For this review, take the finished solid that the model builds, in its own axes (mm). A direction names the side the tool comes from. Round coordinates to 2 decimals unless told otherwise and drop trailing zeros. Write each loop counter-clockwise with the first axis right and the second up, starting at its lowest first coordinate (ties: lowest second). Pieces come first, ordered by that corner, then holes.
Autodesk Inventor part; units mm, degrees
ref_plane "YZ Plane" through (0, 0, 0) normal (1, 0, 0) x (0, 1, 0)
ref_plane "XZ Plane" through (0, 0, 0) normal (0, 1, 0) x (-1, 0, 0)
ref_plane "XY Plane" through (0, 0, 0) normal (0, 0, 1) x (1, 0, 0)
sketch "Sketch1" plane through (0, 0, 0) normal (0, 1, 0) x (-1, 0, 0)
  line L0 (-71.934, -191.4381) -> (-71.9231, -191.4456)
  line L1 (19.6087, -153.4475) -> (19.6065, -153.4456)
  line L2 (-67.3897, -0.1562) -> (-37.3897, -0.1562)
  line L3 (-37.3897, 1.8438) -> (-67.3897, 1.8438)
  line L4 (-62.3897, -3.1562) -> (-42.3897, -3.1562)
  line L5 (-42.3897, -5.1562) -> (-62.3897, -5.1562)
  line L6 (-113.9275, -186.1817) -> (-113.9275, -186.2664)
  line L7 (-115.4443, -311.1974) -> (-115.4443, -311.1982)
  line L8 (-113.9275, -180.4456) -> (-113.9275, -180.5089)
  circle A0 centre (-110.3897, -10.1562) radius 3
  arc A1 (10.8743, -2.1562) -> (10.8743, -18.1562) centre (10.8743, -10.1562) ccw
  arc A2 (-42.3897, -5.1562) -> (-42.3897, -3.1562) centre (-42.3897, -4.1562) ccw
  arc A3 (-62.3897, -3.1562) -> (-62.3897, -5.1562) centre (-62.3897, -4.1562) ccw
  arc A4 (-67.3897, 1.8438) -> (-67.3897, -0.1562) centre (-67.3897, 0.8438) ccw
  arc A5 (-37.3897, -0.1562) -> (-37.3897, 1.8438) centre (-37.3897, 0.8438) ccw
  arc A6 (-104.3897, 9.8438) -> (-104.3897, -30.1562) centre (-104.3897, -10.1562) ccw
  line L9 (5.6103, 9.8438) -> (11.6725, 6.3438)
  line L10 (11.6725, 6.3438) -> (15.6725, 6.3438)
  line L11 (15.6725, 6.3438) -> (15.6725, -0.2278)
  line L12 (15.6725, -0.2278) -> (13.3743, -2.1562)
  line L13 (13.3743, -2.1562) -> (10.8743, -2.1562)
  line L14 (5.6103, 9.8438) -> (-104.3897, 9.8438)
  line L15 (-89.3897, 0.552) -> (-101.3897, 0.552)
  line L16 (-101.3897, 0.552) -> (-95.3897, -6.1562)
  line L17 (-95.3897, -6.1562) -> (-89.3897, 0.552)
  line L18 (-85.3897, -4.1562) -> (-81.3897, -0.1562)
  line L19 (-75.3897, -0.1562) -> (-71.3897, -4.1562)
  line L20 (-71.3897, -4.1562) -> (-85.3897, -4.1562)
  line L21 (-81.3897, -0.1562) -> (-75.3897, -0.1562)
  line L22 (-68.2196, -182.5089) -> (-68.232, -182.5206)
  line L23 (-104.3897, 9.8438) -> (-104.3897, -30.1562)
  line L24 (-104.3897, -10.1562) -> (10.8743, -10.1562)
  line L25 (-110.3897, -10.1562) -> (-104.3897, -10.1562)
  line L26 (10.8743, -2.1562) -> (10.8743, -18.1562)
  line L27 (5.6103, -30.1562) -> (11.6725, -26.6562)
  line L28 (11.6725, -26.6562) -> (15.6725, -26.6562)
  line L29 (15.6725, -26.6562) -> (15.6725, -20.0845)
  line L30 (15.6725, -20.0845) -> (13.3743, -18.1562)
  line L31 (13.3743, -18.1562) -> (10.8743, -18.1562)
  line L32 (5.6103, -30.1562) -> (-104.3897, -30.1562)
  line L33 (-2.3577, 2.8438) -> (-7.5577, 2.8438)
  line L34 (-7.5577, 2.8438) -> (-7.5577, 4.8438)
  line L35 (-2.3577, 4.8438) -> (-7.5577, 4.8438)
  line L36 (-2.3577, 2.8438) -> (-2.3577, 4.8438)
  line L37 (-12.3577, 2.8438) -> (-17.5577, 2.8438)
  line L38 (-17.5577, 2.8438) -> (-17.5577, 4.8438)
  line L39 (-12.3577, 4.8438) -> (-17.5577, 4.8438)
  line L40 (-12.3577, 2.8438) -> (-12.3577, 4.8438)
  line L41 (-46.7577, -10.1562) -> (-46.7577, 9.8438)
  line L42 (-2.3577, -23.1562) -> (-7.5577, -23.1562)
  line L43 (-7.5577, -23.1562) -> (-7.5577, -25.1562)
  line L44 (-2.3577, -25.1562) -> (-7.5577, -25.1562)
  line L45 (-2.3577, -23.1562) -> (-2.3577, -25.1562)
  line L46 (-12.3577, -23.1562) -> (-17.5577, -23.1562)
  line L47 (-17.5577, -23.1562) -> (-17.5577, -25.1562)
  line L48 (-12.3577, -25.1562) -> (-17.5577, -25.1562)
  line L49 (-12.3577, -23.1562) -> (-12.3577, -25.1562)
  circle A7 centre (3.6423, -25.1562) radius 1.55
  circle A8 centre (3.5423, 4.8438) radius 1.55
  circle A9 centre (-83.7577, 4.8438) radius 1.55
  circle A10 centre (-106.7577, 4.8438) radius 1.55
  circle A11 centre (-83.7577, -25.1562) radius 1.55
  circle A12 centre (-106.7577, -25.1562) radius 1.55
  line L50 (-62.3897, -17.1562) -> (-42.3897, -17.1562)
  line L51 (-42.3897, -15.1562) -> (-62.3897, -15.1562)
  line L52 (-67.3897, -20.1562) -> (-37.3897, -20.1562)
  line L53 (-37.3897, -22.1562) -> (-67.3897, -22.1562)
  arc A13 (-42.3897, -17.1562) -> (-42.3897, -15.1562) centre (-42.3897, -16.1562) ccw
  arc A14 (-62.3897, -15.1562) -> (-62.3897, -17.1562) centre (-62.3897, -16.1562) ccw
  arc A15 (-67.3897, -20.1562) -> (-67.3897, -22.1562) centre (-67.3897, -21.1562) ccw
  arc A16 (-37.3897, -22.1562) -> (-37.3897, -20.1562) centre (-37.3897, -21.1562) ccw
  line L54 (-89.3897, -20.8644) -> (-101.3897, -20.8644)
  line L55 (-101.3897, -20.8644) -> (-95.3897, -14.1562)
  line L56 (-95.3897, -14.1562) -> (-89.3897, -20.8644)
  line L57 (-85.3897, -16.1562) -> (-81.3897, -20.1562)
  line L58 (-75.3897, -20.1562) -> (-71.3897, -16.1562)
  line L59 (-71.3897, -16.1562) -> (-85.3897, -16.1562)
  line L60 (-81.3897, -20.1562) -> (-75.3897, -20.1562)
  line L61 (-29.7577, -1.1562) -> (-9.7577, -1.1562)
  line L62 (-9.7577, -1.1562) -> (-14.7577, -6.1562)
  line L63 (-14.7577, -6.1562) -> (-24.7577, -6.1562)
  line L64 (-24.7577, -6.1562) -> (-29.7577, -1.1562)
  line L65 (-29.7577, -19.1562) -> (-9.7577, -19.1562)
  line L66 (-9.7577, -19.1562) -> (-14.7577, -14.1562)
  line L67 (-14.7577, -14.1562) -> (-24.7577, -14.1562)
  line L68 (-24.7577, -14.1562) -> (-29.7577, -19.1562)
  dimension "d39" = 6
  dimension "d54" = 40
  dimension "d55" = 6
  dimension "d56" = 20
  dimension "d58" = 110
  dimension "d60" = 150
  dimension "d61" = 130
  dimension "d62" = 4
  dimension "d63" = 2.5
  dimension "d64" = 7
  dimension "d65" = 3
  dimension "d70" = 8
  dimension "d74" = 2
  dimension "d75" = 5.2
  dimension "d76" = 2
  dimension "d77" = 5.2
  dimension "d78" = 4.8
  dimension "d79" = 13
  dimension "d80" = 13
  dimension "d81" = 29.2
  dimension "d82" = 3.1
  dimension "d83" = 3.1
  dimension "d84" = 5.9
  dimension "d85" = 6
  dimension "d86" = 15
  dimension "d87" = 15
  dimension "d88" = 3.1
  dimension "d89" = 3.1
  dimension "d90" = 15
  dimension "d91" = 15
  dimension "d92" = 37
  dimension "d93" = 23
  dimension "d94" = 12
  dimension "d95" = 9
  dimension "d96" = 14
  dimension "d97" = 6
  dimension "d99" = 4
  dimension "d100" = 9
  dimension "d101" = 6
  dimension "d102" = 10
  dimension "d103" = 2
  dimension "d104" = 20
  dimension "d105" = 2
  dimension "d106" = 5
  dimension "d108" = 30
  dimension "d109" = 10
  dimension "d110" = 42
  dimension "d111" = 5
  dimension "d112" = 20
  dimension "d113" = 10
  dimension "d114" = 45
  dimension "d115" = 4
  dimension "d116" = 22
extrude "Extrusion1" add sketch "Sketch1" along normal blind 3 contours L2 L41 L4 A3 L5 L24 L23 L14 L3 A4 | L2 A5 L3 L41 L14 L9 L10 L11 L12 L13 A1 L24 L5 A2 L4 | L24 A1 L31 L30 L29 L28 L27 L32 L23 | L23 A6
properties part number "topplate.rev4"
(1) We need section A-A, the plane x = 57. Give the boundary of the cut face in (y, z).
Geometry check:
outline: (0, -30.16) - (3, -30.16) - (3, -22.16) - (0, -22.16) - close; (0, -20.16) - (3, -20.16) - (3, -17.16) - (0, -17.16) - close; (0, -15.16) - (3, -15.16) - (3, -5.16) - (0, -5.16) - close; (0, -3.16) - (3, -3.16) - (3, -0.16) - (0, -0.16) - close; (0, 1.84) - (3, 1.84) - (3, 9.84) - (0, 9.84) - close
(2) For faces 5 (the face through (-14.54, 1.48, -1.18)), 6 (the face through (5, 1, -25.156)), 7 (the face through (-15.672, 1, -23)), list the 3-axis set-ups (+Z, -Z, +X, -X, +Y, -Y) from which the entire face can be reached by the end or side of a thin tool; tool diameter is ignored.
Geometry check:
face 5: -X, +Y, -Y
face 6: +Y, -Y
face 7: +Z, -Z, -X, +Y, -Y
(3) Mouldability with a two-part tool opening along X and no side actions: class faces 1 (the face through (82.28, 1.48, 4.38)), 2 (the face through (-12, 1, -18.156)), 3 (the face through (5, 1, 4.844)), 4 (the face through (-8.6, 1.48, -28.43)) as pulls with the +X half, pulls with the -X half, needs draft (parallel to the pull), parting line crosses it, or undercut.
Geometry check:
face 1: undercut
face 2: needs draft
face 3: undercut
face 4: pulls with the -X half
(4) We need section C-C, the plane x = 94. Give the boundary of the cut face in (y, z).
Geometry check:
outline: (0, -30.16) - (3, -30.16) - (3, -20.86) - (0, -20.86) - close; (0, -15.71) - (3, -15.71) - (3, -4.6) - (0, -4.6) - close; (0, 0.55) - (3, 0.55) - (3, 9.84) - (0, 9.84) - close
(5) We need section B-B, the plane z = -11.5. Give the boundary of the cut face in (x, y).
Geometry check:
outline: (-2.99, 0) - (107.71, 0) - (107.71, 3) - (-2.99, 3) - close; (113.07, 0) - (124.34, 0) - (124.34, 3) - (113.07, 3) - close
(6) For line 1 along Z through (x, y) = (54.5, 0.8); line 2 along Z through (x, y) = (36.5, 0.65); line 3 along X through (y, z) = (2.25, -0.5), list the stretches that pass through material, from the lowest coordinate up.
Geometry check:
line 1: z = -30.16 to -22.16, -20.16 to -17.16, -15.16 to -5.16, -3.16 to -0.16, 1.84 to 9.84
line 2: z = -30.16 to -21.61, -20.7 to 0.39, 1.3 to 9.84
line 3: x = -15.35 to 75.05, 81.73 to 90.33, 100.45 to 121.9
(7) For pin 1 Ø0.6 at (y, z) = (1, 4) entering from +X; pin 2 Ø1.6 at (y, z) = (2, 3.5) entering from +X, all flat-tipped, find the tip position at first contact; note any pin that passes through.
Geometry check:
pin 1: stops at x = 118.81
pin 2: stops at x = 119.71
(8) We need section D-D, the plane y = 2.05. State how many separate pieces and enclosed holes the cut face has, and give its area (3 significant figures).
Geometry check:
separate pieces: 1
enclosed holes: 21
area: 4,560 mm2
